Autodesk Inventor part; units mm, degrees
ref_plane "YZ Plane" through (0, 0, 0) normal (1, 0, 0) x (0, 1, 0)
ref_plane "XZ Plane" through (0, 0, 0) normal (0, 1, 0) x (-1, 0, 0)
ref_plane "XY Plane" through (0, 0, 0) normal (0, 0, 1) x (1, 0, 0)
sketch "Schizzo1" plane through (0, 0, 0) normal (0, 0, 1) x (1, 0, 0)
  line L0 (-25, 0) -> (42.5, 0)
  line L1 (-25, 0) -> (-25, 4)
  line L2 (-25, 4) -> (-15, 4)
  line L3 (-15, 4) -> (-15, 10)
  line L4 (-15, 10) -> (15, 10)
  line L5 (15, 10) -> (15, 0)
  point P0 (0, 0)
  point P1 (0, 0)
  point P2 (15, 4)
  point P3 (42.5, 4)
  point P4 (0, 10)
  dimension "d0" = 8
  dimension "d1" = 10
  dimension "d2" = 20
  dimension "d3" = 30
revolve "Rivoluzione1" add sketch "Schizzo1" angle 360 about axis through (-25, 0, 0) along (1, 0, 0)
chamfer "Smusso1" distance 0.5 angle 45 1 edges at (-25, -4, 0)
thread "Filettatura1"
chamfer "Smusso2" distance 1 angle 45 1 edges at (-15, -10, 0)
sketch "Schizzo2" plane through (15, 0, 0) normal (1, 0, 0) x (0, 0, -1)
  circle A0 centre (0, 0) radius 10
  circle A1 centre (0, 0) radius 10
  line L0 (-8.5, 0) -> (-4.25, 7.3612)
  line L1 (-4.25, 7.3612) -> (4.25, 7.3612)
  line L2 (4.25, 7.3612) -> (8.5, 0)
  line L3 (8.5, 0) -> (4.25, -7.3612)
  line L4 (4.25, -7.3612) -> (-4.25, -7.3612)
  line L5 (-4.25, -7.3612) -> (-8.5, 0)
  point P0 (0, 0)
  point P1 (0, 0)
  point P2 (-10, 0)
  dimension "d17" = 17
extrude "Estrusione2" cut sketch "Schizzo2" against normal blind 8
properties part number "Albero cuscinetto"
CAD build for the part. Positions are in the model's coordinates, mm. A direction names the side the tool comes from. Round coordinates to 2 decimals unless told otherwise and drop trailing zeros. Write each loop counter-clockwise with the first axis right and the second up, starting at its lowest first coordinate (ties: lowest second). Pieces come first, ordered by that corner, then holes. Notation, with made-up numbers: M 82,38.25 L 132,38.25 A32 cw 132,76.25 Z; hole C -1.75,-35.75 d4. An arc over 180 degrees is marked long. One line per question, with ' | ' between items.
1. Which spindle directions (+Z, -Z, +X, -X, +Y, -Y) get a long thin tool onto all of the face, cutting with end or side? Do faces 1 (the flat face through (11.056, 3.629, 6.405)), 2 (the cylindrical face through (-19.684, -0.867, -3.905)), 3 (the flat face through (11.056, -3.732, 6.345)). Say none if no direction does.
Working result:
face 1: +Z, +X, +Y | face 2: -X | face 3: +Z, +X, -Y
2. Probe L1, parallel to X at y = 2, z = 4.5; L2, parallel to X at y = 8.5, z = -0.5; L3, parallel to Z at x = -7.5, y = 0. List the from-to ranges inside material, lowest first. Write a range as from..to.
Working result:
L1: -15..15 | L2: -15..7 | L3: -10..10
3. Pin check, flat tips, straight feed: pin 1 Ø6 at (x, y) = (-4, 5) entering from -Z; pin 2 Ø1 at (x, z) = (6.5, -3.5) entering from +Y; pin 3 Ø2 at (x, y) = (6, 2.5) entering from -Z. Stop position of each tip, or through.
Working result:
pin 1: z = -9.8 | pin 2: y = 9.54 | pin 3: z = -9.89
4. Cut at D-D on x = 12.5. Write the cut outline in (y, z), and give its area (3 significant figures).
Working result:
outline: M -7.36,-4.25 L 0,-8.5 L 7.36,-4.25 L 7.36,4.25 L 0,8.5 L -7.36,4.25 Z | area: 188 mm2
5. Cut at A-A on z = 0. Write the cut outline in (x, y).
Working result:
outline: M -25,-3.5 L -24.5,-4 L -15,-4 L -15,-9 L -14,-10 L 7,-10 L 7,-7.36 L 15,-7.36 L 15,7.36 L 7,7.36 L 7,10 L -14,10 L -15,9 L -15,4 L -24.5,4 L -25,3.5 Z
6. Cut at B-B on x = -12.5. Write the cut outline in (y, z), and give its area (3 significant figures).
Working result:
outline: C 0,0 d20 | area: 314 mm2
7. Cut at C-C on x = -19. Write the cut outline in (y, z), and give its area (3 significant figures).
Working result:
outline: C 0,0 d8 | area: 50.3 mm2
